The model under review builds one solid part; all positions refer to its coordinate system, in mm. Face numbers are marked on the shaded views. A direction names the side the tool comes from. Coordinates: 2 decimals unless noted, no trailing zeros. Loops run counter-clockwise (first coordinate to the right, second up) from the corner with the lowest first, then second, coordinate; pieces in that order, holes last. Notation, with made-up numbers: (27.5, 53.25) - (59.5, 53.25) arc R10 cw to (59.5, 70.25) - close; hole circle Ø3 at (51, 47.5). An arc over 180 degrees is marked (long way). One line per item, written item: value. Start each with the question number.
1. Insertion check: P1, Ø8, axis at x = 9, z = 4.5, coming from the -Y side; P2, Ø3, axis at x = 5.5, z = -2, coming from the +Y side; P3, Ø1, axis at y = -10.5, z = 5, coming from the +X side; P4, Ø1.5, axis at y = 10.5, z = -2, coming from the +X side. Each pin has a flat end and moves straight along its axis. Give the tip position at first contact, or say it passes through.
2. To check wall thickness, follow line 1 (Z direction, x = 18.5, y = -2); line 2 (Y direction, x = 15, z = 2.25); line 3 (Z direction, x = 43.5, y = 3.75). State the ranges of each line that lie inside material, in increasing order.
3. Mouldability with a two-part tool opening along Y and no side actions: class the marked faces 1, 2, 3 and 4 as +Y half, -Y half, draft (parallel to the pull), parting line (faces both ways), or undercut.
4. We need section A-A, the plane z = 4. Give the boundary of the cut face in (x, y).
5. We need section B-B, the plane x = 16.5. Give the boundary of the cut face in (y, z), then the cut area to 3 significant figures.
6. For the marked faces 5, 6 and 7, list the 3-axis set-ups (+Z, -Z, +X, -X, +Y, -Y) from which the entire face can be reached by the end or side of a thin tool; tool diameter is ignored.
7. We need section D-D, the plane z = -2.25. Give the boundary of the cut face in (x, y), then the cut area to 3 significant figures.
8. We need section C-C, the plane y = -3.25. Give the boundary of the cut face in (x, z), then the cut area to 3 significant figures.
from build123d import *

# Parameters (mm, degrees)
BOSS_EXTRU_1_DEPTH      = 1.3
ESQUISSE2_W             = 8
ESQUISSE2_H             = 7
BOSS_EXTRU_3_DEPTH      = 4
ESQUISSE5_W             = 5
ESQUISSE5_H             = 8
BOSS_EXTRU_4_DEPTH      = 6
ESQUISSE6_W             = 3
ESQUISSE6_H             = 6
ENL_V_MAT_EXTRU_1_DEPTH = 7
ESQUISSE7_W             = 5
ESQUISSE7_H             = 7
ENL_V_MAT_EXTRU_2_DEPTH = 4
ESQUISSE8_W             = 20
ESQUISSE8_H             = 1.959214555
BOSS_EXTRU_5_DEPTH      = 7.3
BOSS_EXTRU_6_DEPTH      = 1


with BuildPart() as part:
    # Esquisse1 → Boss.-Extru.1 (new body)
    with BuildSketch(Plane.XY):
        Polygon((0, -14.15), (0, 14.15), (20, 14.15), (21.5, 12.65), (60.8, 12.65), (60.8, -12.65), (21.5, -12.65), (20, -14.15), align=None)
    extrude(amount=BOSS_EXTRU_1_DEPTH)

    # Esquisse2 → Boss.-Extru.3 (add)
    with BuildSketch(Plane(origin=(0, 0, 0), x_dir=(-1, 0, 0), z_dir=(0, 0, -1))):
        with Locations((-4, 4.65)):
            Rectangle(ESQUISSE2_W, ESQUISSE2_H)
    extrude(amount=BOSS_EXTRU_3_DEPTH)

    # Esquisse5 → Boss.-Extru.4 (add)
    with BuildSketch(Plane(origin=(0, 0, 0), x_dir=(-1, 0, 0), z_dir=(0, 0, -1))):
        with Locations((-2.5, -6.15)):
            Rectangle(ESQUISSE5_W, ESQUISSE5_H)
    extrude(amount=BOSS_EXTRU_4_DEPTH)

    # Esquisse6 → Enlèv. mat.-Extru.1 (cut)
    with BuildSketch(Plane.ZY):
        with Locations((-2, 4.65)):
            Rectangle(ESQUISSE6_W, ESQUISSE6_H)
    extrude(amount=-ENL_V_MAT_EXTRU_1_DEPTH, mode=Mode.SUBTRACT)

    # Esquisse7 → Enlèv. mat.-Extru.2 (cut)
    with BuildSketch(Plane.ZY):
        with Locations((-3, -6.15)):
            Rectangle(ESQUISSE7_W, ESQUISSE7_H)
    extrude(amount=-ENL_V_MAT_EXTRU_2_DEPTH, mode=Mode.SUBTRACT)

    # Esquisse8 → Boss.-Extru.5 (add)
    with BuildSketch(Plane.XY.offset(1.3)):
        with Locations((10.5, 11.170392723)):
            Rectangle(ESQUISSE8_W, ESQUISSE8_H)
        with Locations((10.5, -11.170392723)):
            Rectangle(ESQUISSE8_W, ESQUISSE8_H)
    extrude(amount=BOSS_EXTRU_5_DEPTH)

    # Esquisse10 → Boss.-Extru.6 (add)
    with BuildSketch(Plane.XY.offset(8.6)):
        Polygon((0.5, 12.15), (0.5, -12.15), (20.5, -12.15), (26.940302788, -4.5), (26.940302788, 4.5), (20.5, 12.15), align=None)
    extrude(amount=BOSS_EXTRU_6_DEPTH)


solid = part.part
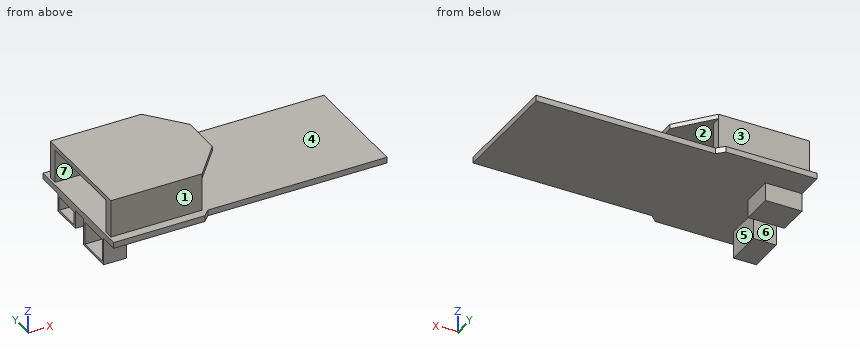
Findings below:
1. P1: y = -14.15
1. P2: y = 8.15
1. P3: x = 20.5
1. P4: through
2. line 1: 0 to 1.3, 8.6 to 9.6
2. line 2: -12.15 to -10.19, 10.19 to 12.15
2. line 3: 0 to 1.3
3. face 1: -Y half
3. face 2: undercut
3. face 3: +Y half
3. face 4: undercut
4. outline: (0.5, -12.15) - (20.5, -12.15) - (20.5, -10.19) - (0.5, -10.19) - close; (0.5, 10.19) - (20.5, 10.19) - (20.5, 12.15) - (0.5, 12.15) - close
5. outline: (-14.15, 0) - (14.15, 0) - (14.15, 1.3) - (12.15, 1.3) - (12.15, 9.6) - (-12.15, 9.6) - (-12.15, 1.3) - (-14.15, 1.3) - close; hole (-10.19, 1.3) - (10.19, 1.3) - (10.19, 8.6) - (-10.19, 8.6) - close
5. area: 89.7 mm2
6. face 5: -Z, +X, -Y
6. face 6: -Z, +X, -X
6. face 7: +X, -X
7. outline: (0, -10.15) - (5, -10.15) - (5, -2.15) - (0, -2.15) - (0, -2.65) - (4, -2.65) - (4, -9.65) - (0, -9.65) - close; (0, 1.15) - (8, 1.15) - (8, 8.15) - (0, 8.15) - (0, 7.65) - (7, 7.65) - (7, 1.65) - (0, 1.65) - close
7. area: 26.0 mm2
8. outline: (0, -6) - (5, -6) - (5, 0) - (60.8, 0) - (60.8, 1.3) - (0, 1.3) - (0, -0.5) - (4, -0.5) - (4, -5.5) - (0, -5.5) - close; (0.5, 8.6) - (26.94, 8.6) - (26.94, 9.6) - (0.5, 9.6) - close
8. area: 115 mm2
